CAD build for the part. Positions are in the model's coordinates, mm. Face numbers are marked on the shaded views. A direction names the side the tool comes from. Round coordinates to 2 decimals unless told otherwise and drop trailing zeros. Order: outer loops, then holes, each group sorted by start corner. A loop starts at its lowest first (then second) coordinate and runs counter-clockwise, first axis right, second up. Notation, with made-up numbers: M -10.5,-13 L 15.5,-13 A24 ccw 15.5,26 Z; hole C 85.5,51 d7. An arc over 180 degrees is marked long. Answer as a JSON object with one key per item and string values.
```python
from build123d import *

# Parameters (mm, degrees)
BASEHEAD_DEPTH     = 2.8
SKETCH6_R          = 2.85
CUT_EXTRUDE1_DEPTH = 1
CUT_EXTRUDE2_DEPTH = 0.386
CIRPATTERN2_COUNT  = 2
CIRPATTERN2_ANGLE  = 90
LPATTERN10_COUNT   = 43
LPATTERN10_PITCH   = 0.3246


with BuildPart() as part:
    # Sketch2 → BaseHead (new body)
    with BuildSketch(Plane(origin=(0, 0, 0), x_dir=(0, 0, -1), z_dir=(1, 0, 0))):
        Polygon((2.020725942, -3.5), (4.041451884, 0), (2.020725942, 3.5), (-2.020725942, 3.5), (-4.041451884, 0), (-2.020725942, -3.5), align=None)
    extrude(amount=BASEHEAD_DEPTH)

    # Sketch10 → Revolve1 (revolve)
    with BuildSketch(Plane(origin=(0, 0, 0), x_dir=(1, 0, 0), z_dir=(0, 1, 0)), mode=Mode.PRIVATE) as revolve1_sk:
        with BuildLine():
            Line((2.8, 2.35), (2.8, 0))
            Line((2.8, 0), (18.8, 0))
            Line((18.8, 0), (18.8, 2))
            Line((18.8, 2), (4.9, 2))
            Line((4.9, 2), (3.966987298, 1.75))
            Line((3.966987298, 1.75), (3.4, 1.75))
            ThreePointArc((3.4, 1.75), (2.975735931, 1.925735931), (2.8, 2.35))
        make_face()
    revolve(revolve1_sk.sketch.rotate(Axis((0, 0, 0), (1, 0, 0)), 180), axis=Axis((0, 0, 0), (1, 0, 0)))

    # Sketch5 → HeadChamfer (revolve, cut)
    with BuildSketch(Plane(origin=(0, 0, 0), x_dir=(1, 0, 0), z_dir=(0, 1, 0)), mode=Mode.PRIVATE) as headchamfer_sk:
        Polygon((0, 4.041451884), (0.433653021, 4.041451884), (0, 2.85), align=None)
    revolve(headchamfer_sk.sketch.rotate(Axis((-0.358389262, 0, 0), (1, 0, 0)), 180), axis=Axis((-0.358389262, 0, 0), (1, 0, 0)), mode=Mode.SUBTRACT)

    # Sketch6 → Cut-Extrude1 (cut)
    with BuildSketch(Plane.ZY):
        Circle(SKETCH6_R)
    extrude(amount=-CUT_EXTRUDE1_DEPTH, mode=Mode.SUBTRACT)

    # Sketch7 → Cut-Extrude2 (cut, symmetric)
    with BuildSketch(Plane(origin=(0, 0, 0), x_dir=(1, 0, 0), z_dir=(0, 1, 0))):
        Polygon((2.93, 0), (0.5, 2.518134715), (0.5, -2.518134715), align=None)
    cut_extrude2 = extrude(amount=CUT_EXTRUDE2_DEPTH, both=True, mode=Mode.SUBTRACT)

    # CirPattern2: Cut-Extrude2 ×2 about axis
    cirpattern2_axis = Axis((0, 0, 0), (-1, 0, 0))
    for i in range(1, CIRPATTERN2_COUNT):
        add(cut_extrude2.rotate(cirpattern2_axis, i * CIRPATTERN2_ANGLE / (CIRPATTERN2_COUNT - 1)), mode=Mode.SUBTRACT)

    # Sketch8 → Cut-Revolve10 (revolve, cut)
    with BuildSketch(Plane.XY, mode=Mode.PRIVATE) as cut_revolve10_sk:
        Polygon((18.8, 1.765740128), (18.93525, 2), (18.93525, 2.2705), (18.66475, 2.2705), (18.66475, 2), align=None)
    cut_revolve10 = revolve(cut_revolve10_sk.sketch.rotate(Axis((14.8, 0, 0), (-1, 0, 0)), 270), axis=Axis((14.8, 0, 0), (-1, 0, 0)), mode=Mode.SUBTRACT)

    # LPattern10: Cut-Revolve10 ×43
    with Locations(*[(-i * LPATTERN10_PITCH, 0, 0) for i in range(1, LPATTERN10_COUNT)]):
        add(cut_revolve10, mode=Mode.SUBTRACT)


solid = part.part
```
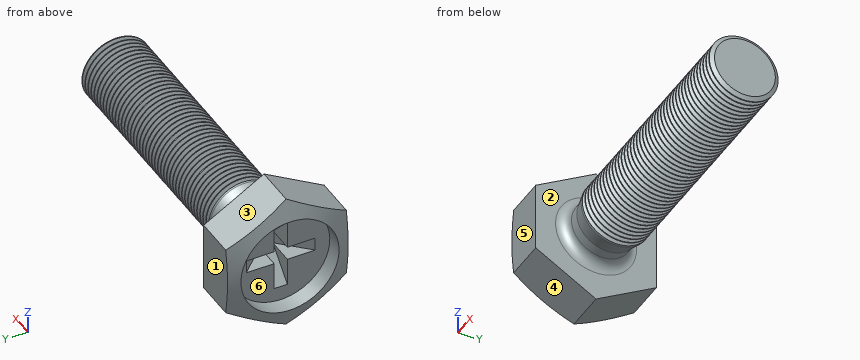
Item 1: Saw through at A-A on x = 1.5. List the corners of the cut face in (y, z).
Worked answers:
{"outline": "M -3.5,-2.02 L 0,-4.04 L 3.5,-2.02 L 3.5,2.02 L 0,4.04 L -3.5,2.02 Z; hole M -1.48,-0.39 L -0.39,-0.39 L -0.39,-1.48 L 0.39,-1.48 L 0.39,-0.39 L 1.48,-0.39 L 1.48,0.39 L 0.39,0.39 L 0.39,1.48 L -0.39,1.48 L -0.39,0.39 L -1.48,0.39 Z"}
Item 2: Wall check: line 1 along Y through (x, z) = (1.5, -1.25); line 2 along Y through (x, z) = (0.7, 0); line 3 along X through (y, z) = (-1.75, 2). Give the ranges that are in metal, low to high. Write a range as [from, to].
Worked answers:
{"line 1": "y = [-3.5, -0.39], [0.39, 3.5]", "line 2": "y = [-3.5, -2.85], [2.85, 3.5]", "line 3": "x = [1, 2.8]"}
Item 3: 3-axis set-ups, long thin cutter, end or side, ignore diameter. For the marked faces 1 and 2: which of +Z, -Z, +X, -X, +Y, -Y reach the whole face in a straight line?
Worked answers:
{"face 1": "+Z, -Z, +X, -X, +Y", "face 2": "+X"}
Item 4: Drop flat-ended pins along their axis: pin 1 Ø1.5 at (x, y) = (17, -0.5) entering from -Z; pin 2 Ø0.5 at (x, y) = (2, -1.5) entering from -Z; pin 3 Ø3 at (y, z) = (-0.5, 2) entering from +X; pin 4 Ø1.7 at (x, y) = (2, -1.5) entering from +Z. Give the stop position or say it passes through.
Worked answers:
{"pin 1": "stops at z = -2", "pin 2": "stops at z = -3.32", "pin 3": "stops at x = 18.8", "pin 4": "stops at z = 3.67"}
Item 5: Two-plate mould, pull along Z, no slides. Class the marked faces 3, 4, 5 and 6: released by +Z, released by -Z, zero draft, split by the parting line, or undercut.
Worked answers:
{"face 3": "released by +Z", "face 4": "released by -Z", "face 5": "zero draft", "face 6": "undercut"}
